Verification items for this drawing (mm, ordinates from the low corner). A direction names the side the tool comes from. Round coordinates to 2 decimals unless told otherwise and drop trailing zeros. Order: outer loops, then holes, each group sorted by start corner. A loop starts at its lowest first (then second) coordinate and runs counter-clockwise, first axis right, second up. Notation, with made-up numbers: M 72.25,64 L 87.25,64 A22 ccw 87.25,71 Z; hole C 78,44 d9. An arc over 180 degrees is marked long. One line per item, written item: value. Start each with the question number.
(1) Cross-section at C-C, the plane z = 26.5. Enter the section's corners in (x, y), and give its area (3 significant figures).
(2) Release check for a two-part mould opening along X. For the marked faces 6, 7 and 8 record: released by +X, released by -X, zero draft, split by the parting line, or undercut.
(3) Cross-section at B-B, the plane x = 15. Enter the section's corners in (y, z).
(4) Access from +Z, -Z, +X, -X, +Y, -Y to the whole of each face (thin tool, end or side, straight path). Record for the marked faces 1, 2, 3, 4 and 5.
(5) Cross-section at A-A, the plane z = 35. Enter the section's corners in (x, y).
(6) Cross-section at D-D, the plane y = 2.5. Enter the section's corners in (x, z), and give its area (3 significant figures).
(7) Thickness scan on L1, parallel to Y at x = 21.05, z = 26; L2, parallel to X at y = 8.25, z = 12.5; L3, parallel to Z at x = 27.5, y = 20.5. Record the ranges inside material, lowest first.
(8) Depth check by flat-ended pin: pin 1 Ø0.8 at (y, z) = (0.5, 1.5) entering from +X; pin 2 Ø4.5 at (x, y) = (15.5, 11) entering from +Z; pin 3 Ø12 at (y, z) = (12, 33) entering from -X. Enter the tip coordinate at first touch or a pass-through.
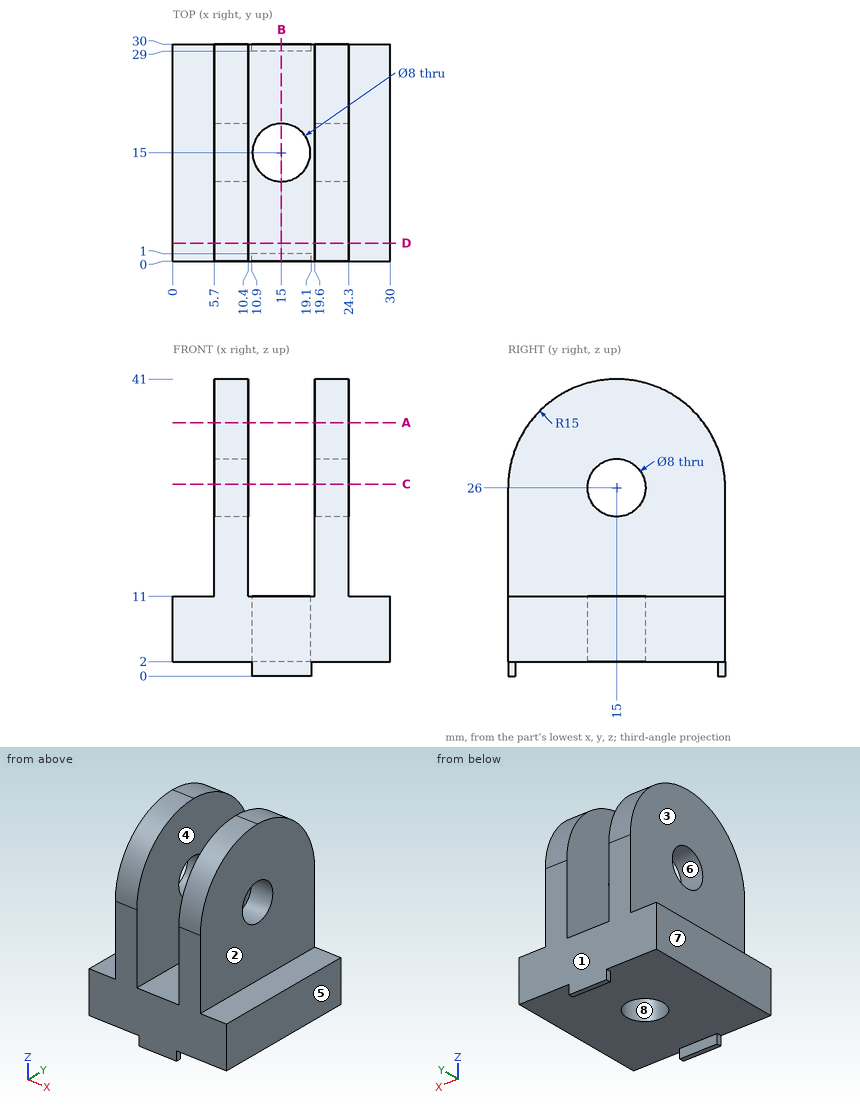
Values found:
1. outline: M 5.7,0.01 L 10.4,0.01 L 10.4,11.03 L 5.7,11.03 Z; M 5.7,18.97 L 10.4,18.97 L 10.4,29.99 L 5.7,29.99 Z; M 19.6,0.01 L 24.3,0.01 L 24.3,11.03 L 19.6,11.03 Z; M 19.6,18.97 L 24.3,18.97 L 24.3,29.99 L 19.6,29.99 Z
1. area: 207 mm^2
2. face 6: zero draft
2. face 7: released by -X
2. face 8: undercut
3. outline: M 0,0 L 1,0 L 1,2 L 11,2 L 11,11 L 0,11 Z; M 19,2 L 29,2 L 29,0 L 30,0 L 30,11 L 19,11 Z
4. face 1: +Z, -Z, +X, -X, +Y
4. face 2: +Z, +X, +Y, -Y
4. face 3: +Z, -X, +Y, -Y
4. face 4: +Z, +Y, -Y
4. face 5: +Z, -Z, +X, +Y, -Y
5. outline: M 5.7,3 L 10.4,3 L 10.4,27 L 5.7,27 Z; M 19.6,3 L 24.3,3 L 24.3,27 L 19.6,27 Z
6. outline: M 0,2 L 30,2 L 30,11 L 24.3,11 L 24.3,34.29 L 19.6,34.29 L 19.6,11 L 10.4,11 L 10.4,34.29 L 5.7,34.29 L 5.7,11 L 0,11 Z
6. area: 489 mm^2
7. L1: 0 to 11, 19 to 30
7. L2: 5.7 to 10.4, 19.6 to 24.3
7. L3: 2 to 11
8. pin 1: x = 19.1
8. pin 2: z = 11
8. pin 3: x = 5.7
